Work out the finished part from the listing and answer in its coordinate system (mm). Round coordinates to 2 decimals unless told otherwise and drop trailing zeros. Order: outer loops, then holes, each group sorted by start corner. A loop starts at its lowest first (then second) coordinate and runs counter-clockwise, first axis right, second up.
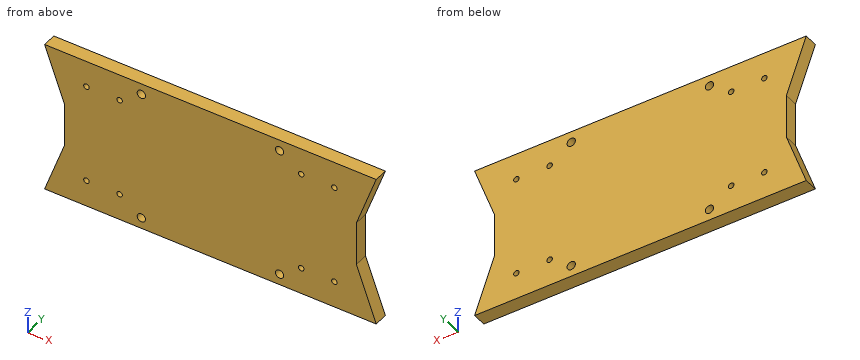
from build123d import *

# Parameters (mm, degrees)
SKETCH1_W           = 67.061286962
SKETCH1_H           = 69.85
SKETCH1_R           = 1.27
BOSS_EXTRUDE1_DEPTH = 6.35
SKETCH2_W           = 20.976278342
SKETCH2_H           = 20.060000012
BOSS_EXTRUDE2_DEPTH = 12.7
BOSS_EXTRUDE3_DEPTH = 6.35
SKETCH4_W           = 170.998259203
SKETCH4_H           = 17.997071231
CUT_EXTRUDE1_DEPTH  = 70.85
SKETCH8_R           = 1.905
CUT_EXTRUDE3_DEPTH  = 13.716


with BuildPart() as part:
    # Sketch1 → Boss-Extrude1 (new body)
    with BuildSketch(Plane(origin=(0, 0, 0), x_dir=(1, 0, 0), z_dir=(0, 1, 0))):
        with Locations((-4.803022, 67.707661351)):
            Rectangle(SKETCH1_W, SKETCH1_H)
        with Locations((3.381343157, 90.407661351)):
            Circle(SKETCH1_R, mode=Mode.SUBTRACT)
        with Locations((18.621343157, 90.407661351)):
            Circle(SKETCH1_R, mode=Mode.SUBTRACT)
        with Locations((3.381343157, 44.947661351)):
            Circle(SKETCH1_R, mode=Mode.SUBTRACT)
        with Locations((18.621343157, 44.947661351)):
            Circle(SKETCH1_R, mode=Mode.SUBTRACT)
    boss_extrude1 = extrude(amount=BOSS_EXTRUDE1_DEPTH)

    # Sketch2 → Boss-Extrude2 (add)
    with BuildSketch(Plane(origin=(0, 6.35, 0), x_dir=(1, 0, 0), z_dir=(0, 1, 0))):
        with Locations((18.23948231, 67.707661351)):
            Rectangle(SKETCH2_W, SKETCH2_H)
    boss_extrude2 = extrude(amount=BOSS_EXTRUDE2_DEPTH)

    # Sketch3 → Boss-Extrude3 (add)
    with BuildSketch(Plane(origin=(0, 6.35, 0), x_dir=(1, 0, 0), z_dir=(0, 1, 0))):
        Polygon((37.841343157, 102.632661351), (28.727621481, 77.737661357), (28.727621481, 102.632661351), align=None)
        Polygon((28.727621481, 57.677661345), (37.841343157, 32.782661351), (28.727621481, 32.782661351), align=None)
    boss_extrude3 = extrude(amount=-BOSS_EXTRUDE3_DEPTH)

    # Mirror2: Boss-Extrude1, Boss-Extrude2, Boss-Extrude3 across plane
    add(boss_extrude1.mirror(Plane(origin=(-38.333665481, 6.35, -32.782661351), x_dir=(0, 0, 1), z_dir=(1, 0, 0))))
    add(boss_extrude2.mirror(Plane(origin=(-38.333665481, 6.35, -32.782661351), x_dir=(0, 0, 1), z_dir=(1, 0, 0))))
    add(boss_extrude3.mirror(Plane(origin=(-38.333665481, 6.35, -32.782661351), x_dir=(0, 0, 1), z_dir=(1, 0, 0))))

    # Sketch4 → Cut-Extrude1 (cut, through all)
    with BuildSketch(Plane.XY.offset(-32.782661351)):
        with Locations((-47.657786445, 15.348535616)):
            Rectangle(SKETCH4_W, SKETCH4_H)
    extrude(amount=-CUT_EXTRUDE1_DEPTH, mode=Mode.SUBTRACT)

    # Sketch8 → Cut-Extrude3 (cut)
    with BuildSketch(Plane(origin=(0, 6.35, 0), x_dir=(1, 0, 0), z_dir=(0, 1, 0))):
        with Locations((-6.558674119, 97.552661351)):
            Circle(SKETCH8_R)
        with Locations((-6.558674119, 37.862661351)):
            Circle(SKETCH8_R)
        with Locations((-171.91881552, 187.895953706)):
            Circle(SKETCH8_R)
        with Locations((-70.058674119, 97.552661351)):
            Circle(SKETCH8_R)
        with Locations((-70.058674119, 37.862661351)):
            Circle(SKETCH8_R)
    extrude(amount=-CUT_EXTRUDE3_DEPTH, mode=Mode.SUBTRACT)


solid = part.part
Item 1: Find section A-A (y = 1). State how many separate pieces and enclosed holes the cut face has, plus the area to 3 significant figures.
Item 2: Find section B-B (z = -62.5). Write down the section's boundary in (x, y).
Item 3: Given pin 1 (1.5 mm diameter, centred on y = 4, z = -46.5, fed in from -X); pin 2 (1.9 mm diameter, centred on y = 4.5, z = -71, fed in from +X); pin 3 (1.5 mm diameter, centred on y = 5.5, z = -88, fed in from -X), each flat-ended and moving along its own axis, determine where each tip first touches the part or whether it passes through.
Item 4: Find section C-C (z = -49). Write down the section's boundary in (x, y).
Item 5: Find the intervals of material crossed by line 1 along X through (y, z) = (6, -96.5); line 2 along X through (y, z) = (3.25, -38); line 3 along Z through (x, y) = (-8, 5.75), in increasing order.
Model answer:
1. separate pieces: 1
1. enclosed holes: 12
1. area: 9,740 mm2
2. outline: (-105.39, 0) - (28.73, 0) - (28.73, 6.35) - (-105.39, 6.35) - close
3. pin 1: stops at x = -109.76
3. pin 2: stops at x = 28.73
3. pin 3: stops at x = -109.43
4. outline: (-108.57, 0) - (31.9, 0) - (31.9, 6.35) - (-108.57, 6.35) - close
5. line 1: x = -112.26 to -71.65, -68.47 to -8.15, -4.97 to 35.6
5. line 2: x = -112.6 to -71.96, -68.16 to -8.46, -4.66 to 35.93
5. line 3: z = -102.63 to -98.8, -96.31 to -39.11, -36.62 to -32.78
